```python
from build123d import *

# Parameters (mm, degrees)
BOSS_EXTRUDE2_DEPTH = 10
SKETCH2_W           = 20
SKETCH2_H           = 20
BOSS_EXTRUDE3_DEPTH = 10
SKETCH3_W           = 40
SKETCH3_H           = 20
BOSS_EXTRUDE4_DEPTH = 20
SKETCH4_W           = 20
SKETCH4_H           = 30
BOSS_EXTRUDE6_DEPTH = 30


with BuildPart() as part:
    # Sketch1 → Boss-Extrude2 (new body)
    with BuildSketch(Plane(origin=(0, 0, 0), x_dir=(1, 0, 0), z_dir=(0, 1, 0))):
        Polygon((0, 0), (60, 0), (60, 20), (90, 20), (90, 50), (60, 50), (0, 50), align=None)
    extrude(amount=BOSS_EXTRUDE2_DEPTH)

    # Sketch2 → Boss-Extrude3 (add)
    with BuildSketch(Plane(origin=(0, 10, 0), x_dir=(1, 0, 0), z_dir=(0, 1, 0))):
        with Locations((10, 10)):
            Rectangle(SKETCH2_W, SKETCH2_H)
    extrude(amount=BOSS_EXTRUDE3_DEPTH)

    # Sketch3 → Boss-Extrude4 (add)
    with BuildSketch(Plane(origin=(0, 10, 0), x_dir=(1, 0, 0), z_dir=(0, 1, 0))):
        with Locations((38.622423296, 40)):
            Rectangle(SKETCH3_W, SKETCH3_H)
    extrude(amount=BOSS_EXTRUDE4_DEPTH)

    # Sketch4 → Boss-Extrude6 (add)
    with BuildSketch(Plane(origin=(0, 10, 0), x_dir=(1, 0, 0), z_dir=(0, 1, 0))):
        with Locations((10, 35)):
            Rectangle(SKETCH4_W, SKETCH4_H)
    extrude(amount=BOSS_EXTRUDE6_DEPTH)


solid = part.part
```
Geometry check sheet. Reference: the model listing, model coordinates, mm. A direction names the side the tool comes from. Coordinates: 2 decimals unless noted, no trailing zeros. Loops run counter-clockwise (first coordinate to the right, second up) from the corner with the lowest first, then second, coordinate; pieces in that order, holes last.
Item 1: Sectioned sample at D-D, the plane x = 74. Record the boundary of the cut face in (y, z), then the cut area to 3 significant figures.
Item 2: Go/stop test with flat-tipped pins: pin 1 Ø8 at (y, z) = (20.5, -33) entering from +X; pin 2 Ø6 at (x, z) = (6.5, -8.5) entering from +Y; pin 3 Ø9 at (y, z) = (22.5, -24) entering from +X. Record where each tip stops, or that it passes through.
Item 3: Sectioned sample at B-B, the plane y = 13. Record the boundary of the cut face in (x, z).
Item 4: Access from +Z, -Z, +X, -X, +Y, -Y to the whole of each face (thin tool, end or side, straight path). Record for faces 1 (the face through (39, 20, -30)), 2 (the face through (39, 30, -40)), 3 (the face through (10, 30, -20)), 4 (the face through (60, 5, -10)).
Item 5: Thickness scan on line 1 (X direction, y = 19.5, z = -8.5); line 2 (X direction, y = 10.5, z = -34); line 3 (Y direction, x = 76, z = -30.5). Record the ranges inside material, lowest first.
Item 6: Sectioned sample at A-A, the plane x = 55. Record the boundary of the cut face in (y, z).
Item 7: Sectioned sample at C-C, the plane y = 37. Record the boundary of the cut face in (x, z), then the cut area to 3 significant figures.
Check result:
1. outline: (0, -50) - (10, -50) - (10, -20) - (0, -20) - close
1. area: 300 mm2
2. pin 1: stops at x = 58.62
2. pin 2: stops at y = 20
2. pin 3: stops at x = 20
3. outline: (0, -50) - (58.62, -50) - (58.62, -30) - (20, -30) - (20, 0) - (0, 0) - close
4. face 1: +Z, +X, +Y
4. face 2: +Z, -Z, +X, +Y
4. face 3: +Z, +X, -X, +Y
4. face 4: +Z, +X, +Y, -Y
5. line 1: x = 0 to 20
5. line 2: x = 0 to 58.62
5. line 3: y = 0 to 10
6. outline: (0, -50) - (30, -50) - (30, -30) - (10, -30) - (10, 0) - (0, 0) - close
7. outline: (0, -50) - (20, -50) - (20, -20) - (0, -20) - close
7. area: 600 mm2
